from build123d import *

# Parameters (mm, degrees)
SKETCH_1_W      = 26.5
SKETCH_1_H      = 8
EXTRUDE_1_DEPTH = 17
FILLET_1_R      = 0.6
SKETCH_2_R      = 0.4
EXTRUDE_2_DEPTH = 1.6


with BuildPart() as part:
    # 草图1 → 凸台-拉伸1 (new body)
    with BuildSketch(Plane.XY):
        Rectangle(SKETCH_1_W, SKETCH_1_H)
    extrude(amount=EXTRUDE_1_DEPTH)

    # 圆角1
    fillet_1_edges = [part.edges().sort_by_distance(p)[0] for p in [
        (0, 4, 17),
        (-13.25, 0, 17),
        (0, -4, 17),
        (-13.25, 0, 0),
        (0, 4, 0),
        (13.25, 0, 0),
        (0, -4, 0),
        (13.25, 0, 17),
        (-13.25, -4, 8.5),
        (-13.25, 4, 8.5),
        (13.25, 4, 8.5),
        (13.25, -4, 8.5),
    ]]
    fillet(fillet_1_edges, radius=FILLET_1_R)

    # 草图2 → 凸台-拉伸2 (add)
    with BuildSketch(Plane(origin=(0, 0, 0), x_dir=(-1, 0, 0), z_dir=(0, 0, -1))):
        with Locations(Location((11, 0, 0), (0, 0, 180))):
            Circle(SKETCH_2_R)
        with Locations(Location((-11, 0, 0), (0, 0, 180))):
            Circle(SKETCH_2_R)
    extrude(amount=EXTRUDE_2_DEPTH)


solid = part.part
Here's how the part is built. I have some questions about the finished solid (model axes, mm). Coordinates: 2 decimals unless noted, no trailing zeros. Order: outer loops, then holes, each group sorted by start corner. A loop starts at its lowest first (then second) coordinate and runs counter-clockwise, first axis right, second up. Notation, with made-up numbers: M 65.25,15.5 L 100.25,15.5 A25 ccw 100.25,31.5 Z; hole C 52.25,-34.75 d4. An arc over 180 degrees is marked long. Answer as CSV lines item,"result".
Item 1: Imagine slicing it at B-B on y = -1.5. Write out the boundary of the cut face in (x, z).
Results found:
outline,"M -13.25,0.6 A0.6 ccw -12.65,0 L 12.65,0 A0.6 ccw 13.25,0.6 L 13.25,16.4 A0.6 ccw 12.65,17 L -12.65,17 A0.6 ccw -13.25,16.4 Z"
Item 2: If I drill on line 1 (Z direction, x = -0.5, y = 2.75); line 2 (X direction, y = 3.5, z = 9); line 3 (Y direction, x = -7, z = 0.25), over which ranges is the centre line in solid material (lowest first)?
Results found:
line 1,"0 to 17"
line 2,"-13.24 to 13.24"
line 3,"-3.89 to 3.89"
Item 3: We'd pull the mould along X, two halves only. Please class faces 1 (the face through (-13.25, 0, 8)), 2 (the face through (-11.295, -0.27, -0.789)), 3 (the face through (0, 0, 17)), 4 (the face through (10.705, -0.27, -0.789)): +X half, -X half, draft (parallel to the pull), parting line (faces both ways), or undercut.
Results found:
face 1,"-X half"
face 2,"undercut"
face 3,"draft"
face 4,"undercut"
Item 4: For pin 1 (2 mm diameter, centred on x = -4.5, y = -0.5, fed in from -Z), with a flat end and sliding along its axis, tell me the tip position at first contact or that it passes through.
Results found:
pin 1,"z = 0"
Item 5: Imagine slicing it at D-D on y = 0. Write out the boundary of the cut face in (x, z), plus the area to 3 significant figures.
Results found:
outline,"M -13.25,0.6 A0.6 ccw -12.65,0 L -11.4,0 L -11.4,-1.6 L -10.6,-1.6 L -10.6,0 L 10.6,0 L 10.6,-1.6 L 11.4,-1.6 L 11.4,0 L 12.65,0 A0.6 ccw 13.25,0.6 L 13.25,16.4 A0.6 ccw 12.65,17 L -12.65,17 A0.6 ccw -13.25,16.4 Z"
area,"453 mm2"
Item 6: Imagine slicing it at A-A on x = -3.5. Write out the boundary of the cut face in (y, z).
Results found:
outline,"M -4,0.6 A0.6 ccw -3.4,0 L 3.4,0 A0.6 ccw 4,0.6 L 4,16.4 A0.6 ccw 3.4,17 L -3.4,17 A0.6 ccw -4,16.4 Z"
Item 7: Imagine slicing it at C-C on x = 11. Write out the boundary of the cut face in (y, z), plus the area to 3 significant figures.
Results found:
outline,"M -4,0.6 A0.6 ccw -3.4,0 L -0.4,0 L -0.4,-1.6 L 0.4,-1.6 L 0.4,0 L 3.4,0 A0.6 ccw 4,0.6 L 4,16.4 A0.6 ccw 3.4,17 L -3.4,17 A0.6 ccw -4,16.4 Z"
area,"137 mm2"
